from build123d import *

# Parameters (mm, degrees)
ESQUISSE2_W             = 50
ESQUISSE2_H             = 50
BOSS_EXTRU_2_DEPTH      = 45
ESQUISSE4_W             = 44
ESQUISSE4_H             = 44
ENL_V_MAT_EXTRU_3_DEPTH = 45
ESQUISSE5_W             = 25
ESQUISSE5_H             = 3
ENL_V_MAT_EXTRU_4_DEPTH = 57
ESQUISSE6_W             = 25
ESQUISSE6_H             = 3
ENL_V_MAT_EXTRU_5_DEPTH = 57
ESQUISSE7_W             = 38
ESQUISSE7_H             = 4
ENL_V_MAT_EXTRU_6_DEPTH = 57
ESQUISSE8_W             = 38
ESQUISSE8_H             = 4
ENL_V_MAT_EXTRU_7_DEPTH = 57
CONG_1_R                = 4


with BuildPart() as part:
    # Esquisse2 → Boss.-Extru.2 (new body)
    with BuildSketch(Plane(origin=(0, 0, 0), x_dir=(1, 0, 0), z_dir=(0, 1, 0))):
        with Locations((25, 25)):
            Rectangle(ESQUISSE2_W, ESQUISSE2_H)
    extrude(amount=-BOSS_EXTRU_2_DEPTH)

    # Esquisse4 → Enlèv. mat.-Extru.3 (cut)
    with BuildSketch(Plane(origin=(0, 0, 0), x_dir=(1, 0, 0), z_dir=(0, 1, 0))):
        with Locations((25, 25)):
            Rectangle(ESQUISSE4_W, ESQUISSE4_H)
    extrude(amount=-ENL_V_MAT_EXTRU_3_DEPTH, mode=Mode.SUBTRACT)

    # Esquisse5 → Enlèv. mat.-Extru.4 (cut)
    with BuildSketch(Plane.XY):
        with Locations((25, -1.5)):
            Rectangle(ESQUISSE5_W, ESQUISSE5_H)
    extrude(amount=-ENL_V_MAT_EXTRU_4_DEPTH, mode=Mode.SUBTRACT)

    # Esquisse6 → Enlèv. mat.-Extru.5 (cut)
    with BuildSketch(Plane(origin=(50, 0, 0), x_dir=(0, 0, -1), z_dir=(1, 0, 0))):
        with Locations((25, -1.5)):
            Rectangle(ESQUISSE6_W, ESQUISSE6_H)
    extrude(amount=-ENL_V_MAT_EXTRU_5_DEPTH, mode=Mode.SUBTRACT)

    # Esquisse7 → Enlèv. mat.-Extru.6 (cut)
    with BuildSketch(Plane.XY):
        with Locations((25, -43)):
            Rectangle(ESQUISSE7_W, ESQUISSE7_H)
    extrude(amount=-ENL_V_MAT_EXTRU_6_DEPTH, mode=Mode.SUBTRACT)

    # Esquisse8 → Enlèv. mat.-Extru.7 (cut)
    with BuildSketch(Plane(origin=(50, 0, 0), x_dir=(0, 0, -1), z_dir=(1, 0, 0))):
        with Locations((25, -43)):
            Rectangle(ESQUISSE8_W, ESQUISSE8_H)
    extrude(amount=-ENL_V_MAT_EXTRU_7_DEPTH, mode=Mode.SUBTRACT)

    # Congé1
    cong_1_edges = [part.edges().sort_by_distance(p)[0] for p in [
        (44, -41, -48.5),
        (44, -41, -1.5),
        (6, -41, -1.5),
        (1.5, -41, -6),
        (1.5, -41, -44),
        (6, -41, -48.5),
        (48.5, -41, -44),
        (48.5, -41, -6),
    ]]
    fillet(cong_1_edges, radius=CONG_1_R - 0.0001)  # a hair under: the kernel refuses the full size


solid = part.part
The model under review builds one solid part; all positions refer to its coordinate system, in mm. A direction names the side the tool comes from. Give positions to 0.01 mm unless a question says otherwise; leave off trailing zeros. Write each loop counter-clockwise with the first axis right and the second up, starting at its lowest first coordinate (ties: lowest second). Pieces come first, ordered by that corner, then holes.
1. Tool access review of faces 4 (the flat face through (48, -45, -48)), 5 (the flat face through (12.5, -2, -1)), 6 (the flat face through (49, -2, -37.5)), 7 (the flat face through (3, 0, -2)), 8 (the cylindrical face through (42.859, -42.203, -1.521)): name each direction out of +Z, -Z, +X, -X, +Y, -Y from which nothing blocks a thin tool from reaching the whole face with its end or side.
2. Wall thickness on L1, parallel to Z at x = 11.5, y = -9.5; L2, parallel to X at y = -14, z = -33.5; L3, parallel to Y at x = 48, z = -17.5: over which ranges is each line inside the solid? List them lowest first.
3. Draft analysis for pull direction X (two halves, no side actions). For faces 1 (the flat face through (25, -22, -47)), 2 (the flat face through (49, -3, -25)), 3 (the flat face through (50, -22, -25)), state which applies: +X half, -X half, draft (parallel to the pull), parting line (faces both ways), or undercut.
4. Add section C-C, the plane y = -6.5. Write out the cut boundary in (x, z), plus the area to 3 significant figures.
5. Add section A-A, the plane z = -24. Write out the cut boundary in (x, y).
6. For P1, Ø0.9, axis at x = 20, z = -48.5, coming from the +Y side; P2, Ø2.5, axis at x = 49, z = -21.5, coming from the -Y side, all flat-tipped, find the tip position at first contact; note any pin that passes through.
7. Add section B-B, the plane x = 21. Write out the cut boundary in (y, z), plus the area to 3 significant figures.
Worked answers:
1. face 4: +Z, -Z, +X, -X, -Y
1. face 5: +Z, -Z, +Y
1. face 6: +X, -X, +Y
1. face 7: +Z, -Z, +X, -X, +Y
1. face 8: +Z, -Z, -Y
2. L1: z = -50 to -47, -3 to 0
2. L2: x = 0 to 3, 47 to 50
2. L3: y = -41 to -3
3. face 1: undercut
3. face 2: draft
3. face 3: +X half
4. outline: (0, -50) - (50, -50) - (50, 0) - (0, 0) - close; hole (3, -47) - (47, -47) - (47, -3) - (3, -3) - close
4. area: 564 mm2
5. outline: (0, -41) - (3, -41) - (3, -3) - (0, -3) - close; (47, -41) - (50, -41) - (50, -3) - (47, -3) - close
6. P1: stops at y = -3
6. P2: stops at y = -41
7. outline: (-41, -50) - (-3, -50) - (-3, -47) - (-41, -47) - close; (-41, -3) - (-3, -3) - (-3, 0) - (-41, 0) - close
7. area: 228 mm2
